CAD build for the part. Positions are in the model's coordinates, mm. Give positions to 0.01 mm unless a question says otherwise; leave off trailing zeros. Loops run counter-clockwise (first coordinate to the right, second up) from the corner with the lowest first, then second, coordinate; pieces in that order, holes last. Notation, with made-up numbers: M 29,-7 L 78,-7 A24 ccw 78,4 Z; hole C 70,-28 d11. An arc over 180 degrees is marked long. Answer as CSV lines item,"result".
```python
from build123d import *

# Parameters (mm, degrees)
F1_DEPTH = 3.175
F3_DEPTH = 3.175


# Not quite as in the source:
# - a feature names something its author has since deleted; it is built from what else it names


with BuildPart() as f1:
    # F0 (on Front) → F1 (new body)
    with BuildSketch(Plane.XZ):
        with BuildLine():
            Line((0, 63.5), (0, 0))
            Line((0, 0), (38.1, 0))
            ThreePointArc((38.1, 0), (60.5506403027, 9.2993596973), (69.85, 31.75))
            ThreePointArc((69.85, 31.75), (60.5506403027, 54.2006403027), (38.1, 63.5))
            Line((38.1, 63.5), (0, 63.5))
        make_face()
        with BuildLine():
            ThreePointArc((60.0519230645, 50.0432692204), (64.9682603323, 41.4776519117), (66.675, 31.75))
            ThreePointArc((66.675, 31.75), (64.9682603323, 22.0223480883), (60.0519230645, 13.4567307796))
            ThreePointArc((60.0519230645, 13.4567307796), (9.525, 31.75), (60.0519230645, 50.0432692204))
        make_face(mode=Mode.SUBTRACT)
        with BuildLine():
            ThreePointArc((55.1737179391, 17.5219017175), (58.997535814, 24.1840485131), (60.325, 31.75))
            ThreePointArc((60.325, 31.75), (58.997535814, 39.3159514869), (55.1737179391, 45.9780982825))
            ThreePointArc((55.1737179391, 45.9780982825), (15.875, 31.75), (55.1737179391, 17.5219017175))
        make_face()
        with BuildLine():
            ThreePointArc((55.1737179391, 45.9780982825), (55.5802350328, 50.4497863142), (60.0519230645, 50.0432692204))
            ThreePointArc((60.0519230645, 50.0432692204), (9.525, 31.75), (60.0519230645, 13.4567307796))
            ThreePointArc((60.0519230645, 13.4567307796), (55.5802350328, 13.0502136858), (55.1737179391, 17.5219017175))
            ThreePointArc((55.1737179391, 17.5219017175), (15.875, 31.75), (55.1737179391, 45.9780982825))
        make_face()
    extrude(amount=F1_DEPTH)

    # F2 (on face) → F3 (cut)
    with BuildSketch(Plane(origin=(0, 0, 0), x_dir=(-1, 0, 0), z_dir=(0, 1, 0))):
        with BuildLine():
            ThreePointArc((-34.1376, 31.75), (-37.3126, 34.925), (-40.4876, 31.75))
            ThreePointArc((-40.4876, 31.75), (-37.3126, 28.575), (-34.1376, 31.75))
        make_face()
    extrude(amount=-F3_DEPTH, mode=Mode.SUBTRACT)


solid = f1.part
```
Q1. Pin check, flat tip, straight feed: P1, Ø10, axis at x = 13.5, z = 40.5, coming from the +Y side. Stop position of the tip, or through.
Solution:
P1,"stops at y = 0"
Q2. Cut at A-A (z = 19). Write the cut outline in (x, y) (3 decimals), and give its area (3 significant figures).
Solution:
outline,"M 0,-3.175 L 56.304,-3.175 L 56.304,0 L 0,0 Z; M 63.673,-3.175 L 67.177,-3.175 L 67.177,0 L 63.673,0 Z"
area,"190 mm²"
Q3. Mould opens along Z. For faces 1 (the cylindrical face through (55.527, -1.565, 50.405)), 2 (the flat face through (19, -2, 0)), 3 (the flat face through (19, -2, 63.5)), 4 (the flat face through (27, -3.175, 32)) say: released by +Z, released by -Z, zero draft, split by the parting line, or undercut.
Solution:
face 1,"undercut"
face 2,"released by -Z"
face 3,"released by +Z"
face 4,"zero draft"
Q4. Wall check: line 1 (X direction, y = -0.85, z = 31.5); line 2 (X direction, y = -2.9, z = 34); line 3 (Z direction, x = 39, y = -2.2). Give the ranges that are in metal, low to high. Write a range as [from, to].
Solution:
line 1,"x = [0, 34.15], [40.48, 60.32], [66.67, 69.85]"
line 2,"x = [0, 35.07], [39.55, 60.21], [66.59, 69.77]"
line 3,"z = [0.01, 29.06], [34.44, 63.49]"
Q5. Cut at C-C (y = -1). Write the cut outline in (x, z) (3 decimals), and give its area (3 significant figures).
Solution:
outline,"M 0,0 L 38.1,0 A31.75 ccw 38.1,63.5 L 0,63.5 Z; hole C 37.313,31.75 d6.35; hole M 55.174,17.522 A3.175 ccw 60.052,13.457 A28.575 ccw 60.052,50.043 A3.175 ccw 55.174,45.978 A22.225 cw Z"
area,"3,720 mm²"
Q6. Cut at D-D (z = 36). Write the cut outline in (x, y) (3 decimals).
Solution:
outline,"M 0,-3.175 L 59.915,-3.175 L 59.915,0 L 0,0 Z; M 66.357,-3.175 L 69.564,-3.175 L 69.564,0 L 66.357,0 Z"
Q7. Cut at B-B (x = 58). Write the cut outline in (y, z) (1 decimal), and give its area (3 significant figures).
Solution:
outline,"M -3.2,7 L 0,7 L 0,12.3 L -3.2,12.3 Z; M -3.2,21.9 L 0,21.9 L 0,41.6 L -3.2,41.6 Z; M -3.2,51.2 L 0,51.2 L 0,56.5 L -3.2,56.5 Z"
area,"96.7 mm²"
